Work out the finished part from the listing and answer in its coordinate system (mm). Face numbers are marked on the shaded views. A direction names the side the tool comes from. Round coordinates to 2 decimals unless told otherwise and drop trailing zeros. Loops run counter-clockwise (first coordinate to the right, second up) from the corner with the lowest first, then second, coordinate; pieces in that order, holes last. Notation, with made-up numbers: (29, 11) -> (41, 11) arc R29 cw to (41, 45) -> close; hole circle Ø6 at (50.25, 27). An arc over 180 degrees is marked (long way). Write item = value, one per line. Start each with the question number.
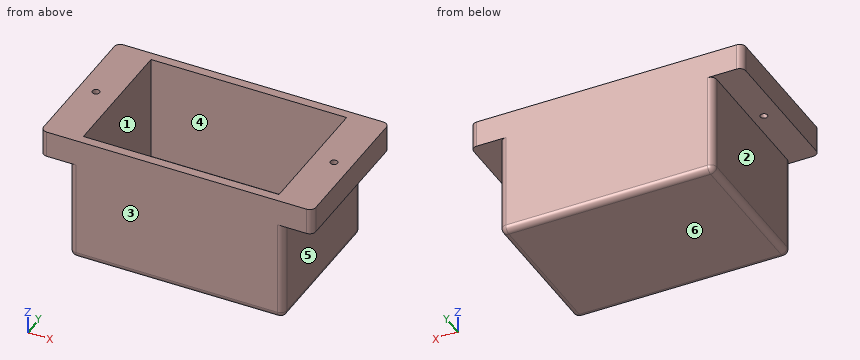
```python
from build123d import *

# Parameters (mm, degrees)
SKETCH1_W                = 133.5
SKETCH1_H                = 73.7
SKETCH1_R                = 1.725
BOSS_EXTRUDE1_DEPTH      = 7.5
BOSS_EXTRUDE1_DEPTH_BACK = 5.5
SKETCH2_W                = 105
SKETCH2_H                = 73.7
BOSS_EXTRUDE2_DEPTH      = 50
SKETCH6_W                = 96
SKETCH6_H                = 65
CUT_EXTRUDE3_DEPTH       = 52
FILLET5_R                = 3
FILLET6_R                = 3


with BuildPart() as part:
    # Sketch1 → Boss-Extrude1 (new body, two sides)
    with BuildSketch(Plane.XY) as boss_extrude1_sk:
        Rectangle(SKETCH1_W, SKETCH1_H)
        with Locations((-58.35, 0)):
            Circle(SKETCH1_R, mode=Mode.SUBTRACT)
        with Locations((58.35, 0)):
            Circle(SKETCH1_R, mode=Mode.SUBTRACT)
    extrude(amount=BOSS_EXTRUDE1_DEPTH)
    extrude(boss_extrude1_sk.sketch, amount=-BOSS_EXTRUDE1_DEPTH_BACK)

    # Sketch2 → Boss-Extrude2 (add)
    with BuildSketch(Plane(origin=(0, 0, -5.5), x_dir=(-1, 0, 0), z_dir=(0, 0, -1))):
        Rectangle(SKETCH2_W, SKETCH2_H)
    extrude(amount=BOSS_EXTRUDE2_DEPTH)

    # Sketch6 → Cut-Extrude3 (cut)
    with BuildSketch(Plane.XY.offset(7.5)):
        Rectangle(SKETCH6_W, SKETCH6_H)
    extrude(amount=-CUT_EXTRUDE3_DEPTH, mode=Mode.SUBTRACT)

    # Fillet5
    fillet5_edges = [part.edges().sort_by_distance(p)[0] for p in [
        (-66.75, 36.85, 1),
        (66.75, 36.85, 1),
        (66.75, -36.85, 1),
        (-66.75, -36.85, 1),
    ]]
    fillet(fillet5_edges, radius=FILLET5_R)

    # Fillet6
    fillet6_edges = [part.edges().sort_by_distance(p)[0] for p in [
        (52.5, 36.85, -30.5),
        (52.5, -36.85, -30.5),
        (-52.5, -36.85, -30.5),
        (-52.5, 36.85, -30.5),
        (52.5, 0, -55.5),
        (0, -36.85, -55.5),
        (-52.5, 0, -55.5),
        (0, 36.85, -55.5),
    ]]
    fillet(fillet6_edges, radius=FILLET6_R)


solid = part.part
```
Item 1: A tool of negligible diameter and unlimited length cuts with its end or side. For the marked faces 4, 5 and 6, from which of +Z, -Z, +X, -X, +Y, -Y can it reach the whole face along a straight path? Write none if from no direction.
Item 2: Section A-A (y = 0) is taken. Determine the outline of the cut face in (x, z) (3 decimals).
Item 3: The mould has two halves that part along X. Classify the marked faces 1, 2 and 3: pulls with the +X half, pulls with the -X half, needs draft (parallel to the pull), parting line crosses it, or undercut.
Item 4: Section C-C (z = -27) is taken. Determine the outline of the cut face in (x, y), then the cut area to 3 significant figures.
Item 5: Section B-B (x = -58.35) is taken. Determine the outline of the cut face in (y, z) (3 decimals), then the cut area to 3 significant figures.
Item 6: Section D-D (y = 30.5) is taken. Determine the outline of the cut face in (x, z), then the cut area to 3 significant figures.
Item 7: Flat-ended cylindrical pins translate along their axes: pin 1 (4.5 mm diameter, centred on x = -58.35, y = 0, fed in from -Z); pin 2 (4.5 mm diameter, centred on x = -58.35, y = 0, fed in from +Z); pin 3 (12 mm diameter, centred on x = -9, y = -20, fed in from +Z); pin 4 (4 mm diameter, centred on x = 53.5, y = -25.5, fed in from -Z). Find the tip coordinate at first contact, or state that the pin passes through.
Item 8: Find the intervals of material crossed by line 1 along Y through (x, z) = (-58.35, -2.8) (3 decimals); line 2 along Y through (x, z) = (46.5, -7); line 3 along X through (y, z) = (30.5, -43.5), in increasing order. Write a range as [from, to].
Worked answers:
q1.face_4 = +Z
q1.face_5 = -Z, +X, +Y, -Y
q1.face_6 = -Z, +X, -X, +Y, -Y
q2.outline = (-66.75, -5.5) -> (-60.075, -5.5) -> (-60.075, 7.5) -> (-66.75, 7.5) -> close; (-56.625, -5.5) -> (-52.5, -5.5) -> (-52.5, -52.5) arc R3 ccw to (-49.5, -55.5) -> (49.5, -55.5) arc R3 ccw to (52.5, -52.5) -> (52.5, -5.5) -> (56.625, -5.5) -> (56.625, 7.5) -> (48, 7.5) -> (48, -44.5) -> (-48, -44.5) -> (-48, 7.5) -> (-56.625, 7.5) -> close; (60.075, -5.5) -> (66.75, -5.5) -> (66.75, 7.5) -> (60.075, 7.5) -> close
q3.face_1 = undercut
q3.face_2 = pulls with the -X half
q3.face_3 = needs draft
q4.outline = (-52.5, -33.85) arc R3 ccw to (-49.5, -36.85) -> (49.5, -36.85) arc R3 ccw to (52.5, -33.85) -> (52.5, 33.85) arc R3 ccw to (49.5, 36.85) -> (-49.5, 36.85) arc R3 ccw to (-52.5, 33.85) -> close; hole (-48, -32.5) -> (48, -32.5) -> (48, 32.5) -> (-48, 32.5) -> close
q4.area = 1,490 mm2
q5.outline = (-36.85, -5.5) -> (-1.725, -5.5) -> (-1.725, 7.5) -> (-36.85, 7.5) -> close; (1.725, -5.5) -> (36.85, -5.5) -> (36.85, 7.5) -> (1.725, 7.5) -> close
q5.area = 913 mm2
q6.outline = (-66.75, -5.5) -> (-52.5, -5.5) -> (-52.5, -52.5) arc R3 ccw to (-49.5, -55.5) -> (49.5, -55.5) arc R3 ccw to (52.5, -52.5) -> (52.5, -5.5) -> (66.75, -5.5) -> (66.75, 7.5) -> (48, 7.5) -> (48, -44.5) -> (-48, -44.5) -> (-48, 7.5) -> (-66.75, 7.5) -> close
q6.area = 1,990 mm2
q7.pin_1 = -5.5
q7.pin_2 = 7.5
q7.pin_3 = -44.5
q7.pin_4 = -54.74
q8.line_1 = [-36.85, -1.725], [1.725, 36.85]
q8.line_2 = [-36.85, -32.5], [32.5, 36.85]
q8.line_3 = [-52.5, -48], [48, 52.5]
